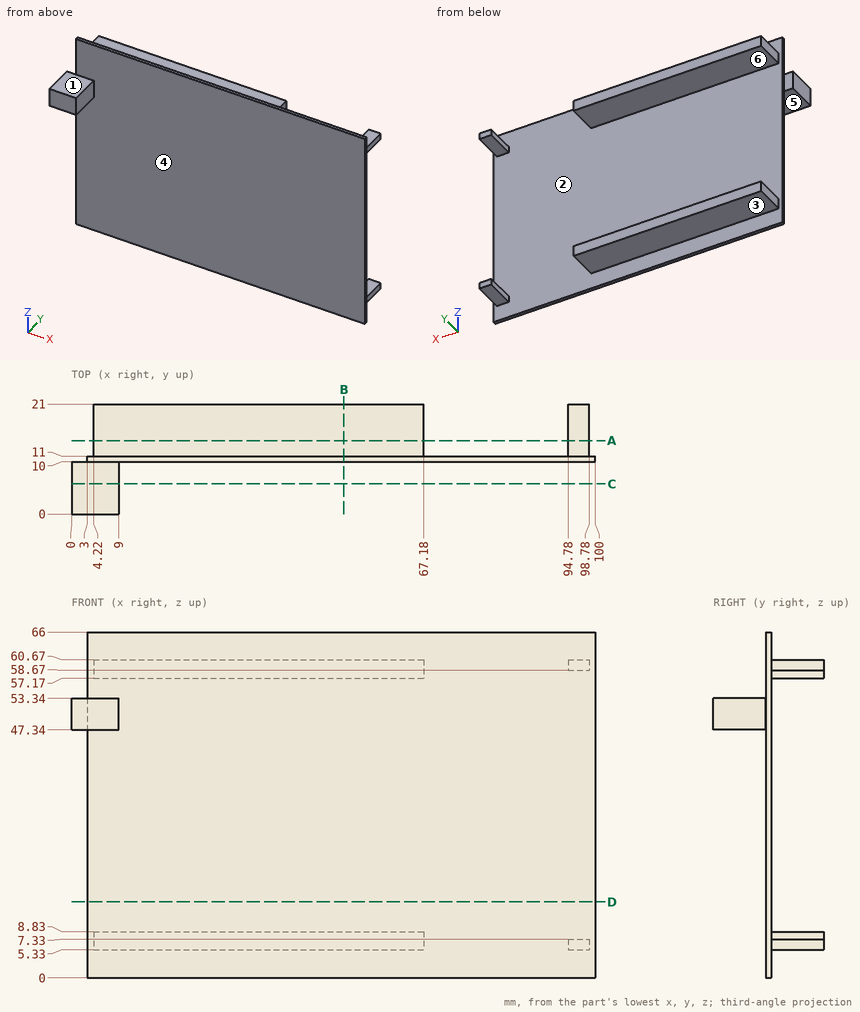
Design review of the part shown in the three views and the two pictorial views. Dimensions are in mm from the part's minimum x, y and z. A direction names the side the tool comes from. Coordinates: 2 decimals unless noted, no trailing zeros. Write each loop counter-clockwise with the first axis right and the second up, starting at its lowest first coordinate (ties: lowest second). Pieces come first, ordered by that corner, then holes.
(1) Add section A-A on y = 14. Give the boundary of the cut face in (x, z).
(2) Add section D-D on z = 14.5. Give the boundary of the cut face in (x, y), then the cut area to 3 significant figures.
(3) For pin 1 Ø12 at (x, z) = (49.5, 58) entering from -Y; pin 2 Ø4 at (y, z) = (18, 7) entering from -X; pin 3 Ø1 at (y, z) = (17, 7.5) entering from +X; pin 4 Ø11 at (x, y) = (35, 16) entering from +Z, all flat-tipped, find the tip position at first contact; note any pin that passes through.
(4) Tool access review of the marked faces 5 and 6: name each direction out of +Z, -Z, +X, -X, +Y, -Y from which nothing blocks a thin tool from reaching the whole face with its end or side.
(5) Add section B-B on x = 52. Give the boundary of the cut face in (y, z).
(6) Add section C-C on y = 5.75. Give the boundary of the cut face in (x, z).
(7) Wall thickness on probe 1 along Z at (x, y) = (47, 13); probe 2 along Y at (x, z) = (66, 9); probe 3 along X at (y, z) = (10.5, 58): over which ranges is each line inside the solid? List them lowest first.
(8) The part is to be moulded in two halves that separate along Z. For the marked faces 1, 2, 3 and 4, say which applies: +Z half, -Z half, draft (parallel to the pull), parting line (faces both ways), or undercut.
Answer sheet:
1. outline: (4.22, 5.33) - (67.18, 5.33) - (67.18, 8.83) - (4.22, 8.83) - close; (4.22, 57.17) - (67.18, 57.17) - (67.18, 60.67) - (4.22, 60.67) - close; (94.78, 5.33) - (98.78, 5.33) - (98.78, 7.33) - (94.78, 7.33) - close; (94.78, 58.67) - (98.78, 58.67) - (98.78, 60.67) - (94.78, 60.67) - close
2. outline: (3, 10) - (100, 10) - (100, 11) - (3, 11) - close
2. area: 97.0 mm2
3. pin 1: stops at y = 10
3. pin 2: stops at x = 4.22
3. pin 3: stops at x = 98.78
3. pin 4: stops at z = 66
4. face 5: -Z, +X, -X, -Y
4. face 6: +X, -X, +Y
5. outline: (10, 0) - (11, 0) - (11, 5.33) - (21, 5.33) - (21, 8.83) - (11, 8.83) - (11, 57.17) - (21, 57.17) - (21, 60.67) - (11, 60.67) - (11, 66) - (10, 66) - close
6. outline: (0, 47.34) - (9, 47.34) - (9, 53.34) - (0, 53.34) - close
7. probe 1: z = 5.33 to 8.83, 57.17 to 60.67
7. probe 2: y = 10 to 11
7. probe 3: x = 3 to 100
8. face 1: +Z half
8. face 2: undercut
8. face 3: -Z half
8. face 4: draft
